The drawing under review shows one solid part. Ordinate dimensions are in mm from its lowest x, y, z. Give positions to 0.01 mm unless a question says otherwise; leave off trailing zeros. Order: outer loops, then holes, each group sorted by start corner. A loop starts at its lowest first (then second) coordinate and runs counter-clockwise, first axis right, second up. Notation, with made-up numbers: (24, 81.25) -> (59, 81.25) arc R19 cw to (59, 87.25) -> close; hole circle Ø2 at (78.5, 13.5). An arc over 180 degrees is marked (long way). Return JSON: item names as keys, results as strings. Group by question number.
1) Add section C-C (x = 35.5). Give the boundary of the cut face in (y, z) (1 decimal).
2) The part is to be moulded in two halves that separate along Y. For the marked faces 1, 2 and 3, say which applies: released by +Y, released by -Y, zero draft, split by the parting line, or undercut.
3) To check wall thickness, follow line 1 along Y through (x, z) = (23.5, 4.05); line 2 along X through (y, z) = (32, 0.9) (1 decimal); line 3 along Y through (x, z) = (22, 1). State the ranges of each line that lie inside material, in increasing order.
4) Insertion check: P1, Ø2.5, axis at x = 38.68, y = 23.5, coming from the +Z side; P2, Ø3, axis at y = 19, z = 3.5, coming from the +X side; P3, Ø3, axis at y = 39, z = 2.5, coming from the +X side (1 decimal). Each pin has a flat end and moves straight along its axis. Give the tip position at first contact, or say it passes through.
5) Add section A-A (y = 23.5). Give the boundary of the cut face in (x, z), then the cut area to 3 significant figures.
6) Add section D-D (z = 2.9). State how many separate pieces and enclosed holes the cut face has, then the cut area to 3 significant figures.
7) Add section B-B (x = 23.5). Give the boundary of the cut face in (y, z), then the cut area to 4 significant figures.
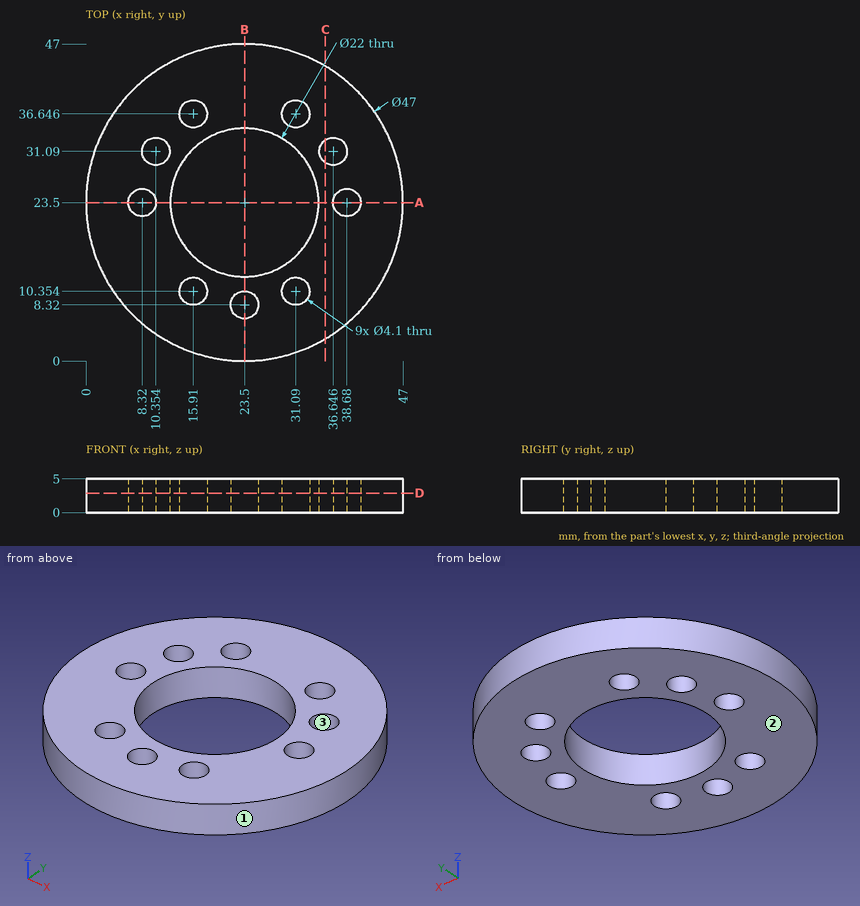
Evaluation:
{
 "1": {"outline": "(3.3, 0) -> (29.4, 0) -> (29.4, 5) -> (3.3, 5) -> close; (32.8, 0) -> (43.7, 0) -> (43.7, 5) -> (32.8, 5) -> close"},
 "2": {"face 1": "split by the parting line", "face 2": "zero draft", "face 3": "undercut"},
 "3": {"line 1": "0 to 6.27, 10.37 to 12.5, 34.5 to 47", "line 2": "1.6 to 8.5, 12.2 to 16.5, 30.5 to 34.8, 38.5 to 45.4", "line 3": "0.05 to 6.92, 9.72 to 12.6, 34.4 to 46.95"},
 "4": {"P1": "through", "P2": "x = 46.81", "P3": "x = 42.4"},
 "5": {"outline": "(0, 0) -> (6.27, 0) -> (6.27, 5) -> (0, 5) -> close; (10.37, 0) -> (12.5, 0) -> (12.5, 5) -> (10.37, 5) -> close; (34.5, 0) -> (36.63, 0) -> (36.63, 5) -> (34.5, 5) -> close; (40.73, 0) -> (47, 0) -> (47, 5) -> (40.73, 5) -> close", "area": "84.0 mm^2"},
 "6": {"separate pieces": "1", "enclosed holes": "10", "area": "1,240 mm^2"},
 "7": {"outline": "(0, 0) -> (6.27, 0) -> (6.27, 5) -> (0, 5) -> close; (10.37, 0) -> (12.5, 0) -> (12.5, 5) -> (10.37, 5) -> close; (34.5, 0) -> (47, 0) -> (47, 5) -> (34.5, 5) -> close", "area": "104.5 mm^2"}
}
